Could you check a few things on this model? Use its own coordinates, in mm. Face numbers are marked on the shaded views. A direction names the side the tool comes from. Coordinates: 2 decimals unless noted, no trailing zeros. Loops run counter-clockwise (first coordinate to the right, second up) from the corner with the lowest first, then second, coordinate; pieces in that order, holes last. Notation, with made-up numbers: (88, 2) -> (139, 2) arc R26 cw to (139, 17) -> close; hole circle Ø5 at (63, -26.75). An arc over 180 degrees is marked (long way). One line per question, with ' | ' between items.
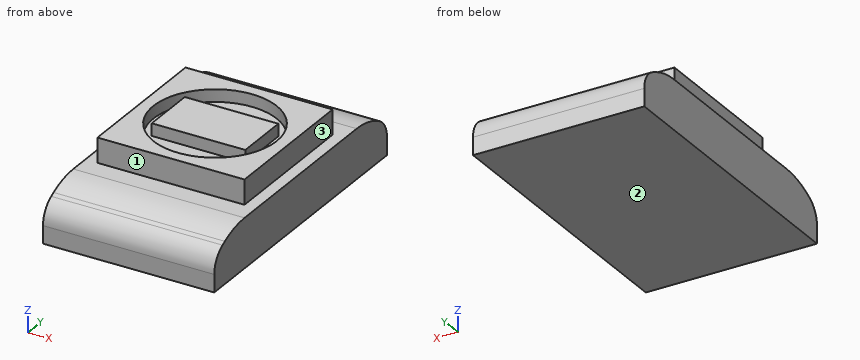
```python
from build123d import *

# Parameters (mm, degrees)
SKETCH1_W           = 6.94
SKETCH1_H           = 9
BOSS_EXTRUDE1_DEPTH = 2
SKETCH3_W           = 6.94
SKETCH3_H           = 1.5
BOSS_EXTRUDE2_DEPTH = 1
SKETCH5_W           = 6.94
SKETCH5_H           = 1.5
BOSS_EXTRUDE3_DEPTH = 1
BOSS_EXTRUDE4_DEPTH = 6.94
FILLET4_R           = 3
FILLET5_R           = 1
FILLET6_R           = 3
FILLET7_R           = 1
SKETCH1_4_W         = 5.96
SKETCH1_4_H         = 5.96
BOSS_EXTRUDE5_DEPTH = 1
SKETCH8_R           = 2.5
CUT_EXTRUDE1_DEPTH  = 0.5
SKETCH8_3_W         = 3.79167841
SKETCH8_3_H         = 2.234967368
BOSS_EXTRUDE6_DEPTH = 0.5


with BuildPart() as part:
    # Sketch1 → Boss-Extrude1 (new body)
    with BuildSketch(Plane.XY):
        Rectangle(SKETCH1_W, SKETCH1_H)
    extrude(amount=-BOSS_EXTRUDE1_DEPTH)

    # Sketch3 → Boss-Extrude2 (add)
    with BuildSketch(Plane(origin=(0, 0.899682646, 1.799761941), x_dir=(-1, 0, 0), z_dir=(0, -0.4471347413551615, -0.8944666137275626))):
        with Locations((0, 4.775099762)):
            Rectangle(SKETCH3_W, SKETCH3_H)
    extrude(amount=BOSS_EXTRUDE2_DEPTH)

    # Sketch5 → Boss-Extrude3 (add)
    with BuildSketch(Plane(origin=(0, -0.880909966, 1.785523027), x_dir=(1, 0, 0), z_dir=(0, -0.4424452173048707, 0.8967955339340434))):
        with Locations((0, -4.785579903)):
            Rectangle(SKETCH5_W, SKETCH5_H)
    extrude(amount=-BOSS_EXTRUDE3_DEPTH)

    # Sketch7 → Boss-Extrude4 (add)
    with BuildSketch(Plane.ZY.offset(3.47)):
        Polygon((-2, 4.5), (-1.117984713, 4.5), (-1.565168726, 5.394565179), (-0.670702112, 5.841699921), (-2, 5.841699921), align=None)
        Polygon((-2, -4.5), (-1.115081378, -4.5), (-1.56046336, -5.402748084), (-0.663667826, -5.845193301), (-2, -5.845193301), align=None)
    extrude(amount=-BOSS_EXTRUDE4_DEPTH)

    # Fillet4
    fillet4_edges = [part.edges().sort_by_distance(p)[0] for p in [
        (0, -4.5, 0),
    ]]
    fillet(fillet4_edges, radius=FILLET4_R)

    # Fillet5
    fillet5_edges = [part.edges().sort_by_distance(p)[0] for p in [
        (0, -5.845193301, -0.663667826),
    ]]
    fillet(fillet5_edges, radius=FILLET5_R)

    # Fillet6
    fillet6_edges = [part.edges().sort_by_distance(p)[0] for p in [
        (0, 4.5, 0),
    ]]
    fillet(fillet6_edges, radius=FILLET6_R)

    # Fillet7
    fillet7_edges = [part.edges().sort_by_distance(p)[0] for p in [
        (0, 5.841699921, -0.670702112),
    ]]
    fillet(fillet7_edges, radius=FILLET7_R)

    # Sketch1<4> → Boss-Extrude5 (add)
    with BuildSketch(Plane.XY):
        Rectangle(SKETCH1_4_W, SKETCH1_4_H)
    extrude(amount=BOSS_EXTRUDE5_DEPTH)

    # Sketch8 → Cut-Extrude1 (cut)
    with BuildSketch(Plane.XY.offset(1)):
        Circle(SKETCH8_R)
    extrude(amount=-CUT_EXTRUDE1_DEPTH, mode=Mode.SUBTRACT)

    # Sketch8<3> → Boss-Extrude6 (add)
    with BuildSketch(Plane.XY.offset(1)):
        Rectangle(SKETCH8_3_W, SKETCH8_3_H)
    extrude(amount=-BOSS_EXTRUDE6_DEPTH)


solid = part.part
```
Q1. For pin 1 (0.5 mm diameter, centred on x = -1, z = 0.5, fed in from -Y); pin 2 (0.6 mm diameter, centred on x = -0.5, z = 1, fed in from +Y); pin 3 (0.5 mm diameter, centred on y = 1, z = 0.5, fed in from +X), each with a flat end and sliding along its axis, tell me the tip position at first contact or that it passes through.
Values follow:
pin 1: stops at y = -2.98 | pin 2: stops at y = 2.98 | pin 3: stops at x = 2.98
Q2. Imagine slicing it at B-B on x = -1.5. Write out the boundary of the cut face in (y, z).
Values follow:
outline: (-5.85, -2) -> (5.84, -2) -> (5.84, -1.29) arc R1 ccw to (5.29, -0.39) -> (5.13, -0.32) arc R3 ccw to (3.79, 0) -> (2.98, 0) -> (2.98, 1) -> (2, 1) -> (2, 0.5) -> (1.12, 0.5) -> (1.12, 1) -> (-1.12, 1) -> (-1.12, 0.5) -> (-2, 0.5) -> (-2, 1) -> (-2.98, 1) -> (-2.98, 0) -> (-3.8, 0) arc R3 ccw to (-5.13, -0.31) -> (-5.29, -0.39) arc R1 ccw to (-5.85, -1.29) -> close
Q3. Imagine slicing it at D-D on y = -2. Write out the boundary of the cut face in (x, z).
Values follow:
outline: (-3.47, -2) -> (3.47, -2) -> (3.47, 0) -> (2.98, 0) -> (2.98, 1) -> (1.5, 1) -> (1.5, 0.5) -> (-1.5, 0.5) -> (-1.5, 1) -> (-2.98, 1) -> (-2.98, 0) -> (-3.47, 0) -> close
Q4. Please list where these lines run through material, in increasing order: L1, parallel to Y at x = 0, z = 0.6; L2, parallel to X at y = -2.75, z = 0.25; L3, parallel to Z at x = 0.75, y = 1.5. Write a range as [from, to].
Values follow:
L1: y = [-2.98, -2.5], [-1.12, 1.12], [2.5, 2.98] | L2: x = [-2.98, 2.98] | L3: z = [-2, 0.5]
Q5. Imagine slicing it at A-A on y = 0. Write out the boundary of the cut face in (x, z).
Values follow:
outline: (-3.47, -2) -> (3.47, -2) -> (3.47, 0) -> (2.98, 0) -> (2.98, 1) -> (2.5, 1) -> (2.5, 0.5) -> (1.9, 0.5) -> (1.9, 1) -> (-1.9, 1) -> (-1.9, 0.5) -> (-2.5, 0.5) -> (-2.5, 1) -> (-2.98, 1) -> (-2.98, 0) -> (-3.47, 0) -> close
Q6. For the marked faces 1, 2 and 3, which set-ups out of +Z, -Z, +X, -X, +Y, -Y let a thin tool reach every point of the face, with its end or its side?
Values follow:
face 1: +Z, +X, -X, -Y | face 2: -Z, +X, -X, +Y, -Y | face 3: +Z, +X, +Y, -Y
Q7. Imagine slicing it at C-C on z = 0.3. Write out the boundary of the cut face in (x, y).
Values follow:
outline: (-2.98, -2.98) -> (2.98, -2.98) -> (2.98, 2.98) -> (-2.98, 2.98) -> close
